Study the drawing (mm; zero at the part's minimum x, y, z) and answer. Coordinates: 2 decimals unless noted, no trailing zeros. Order: outer loops, then holes, each group sorted by start corner. A loop starts at its lowest first (then second) coordinate and runs counter-clockwise, first axis right, second up. Notation, with made-up numbers: (35, 80) -> (65, 80) arc R26 ccw to (65, 116) -> close; hole circle Ø1 at (10.25, -4.75). An arc over 180 degrees is marked (long way). Answer as CSV lines item,"result". Start each with the question number.
Item 1: Section C-C (x = 115) is taken. Write down the section's boundary in (y, z) (1 decimal).
Item 2: Straight lines are drawn through the part: L1, parallel to X at y = 15, z = 3.5; L2, parallel to Y at x = 127.5, z = 1.55 (1 decimal). For each, find the intervals that lie inside material, in ascending order.
Item 3: Section B-B (y = 126) is taken. Write down the section's boundary in (x, z).
Item 4: Each of these flat-tipped pins is pushed along its axis until it touches: pin 1 Ø1.2 at (y, z) = (3, 2.5) entering from +X; pin 2 Ø2 at (x, z) = (173.5, 3) entering from -Y (1 decimal); pin 3 Ø1.3 at (y, z) = (28.5, 3) entering from -X. Where does it stop, or does it pass through?
Item 5: Section A-A (z = 1.5) is taken. Write down the section's boundary in (x, y) (1 decimal), then the cut area to 3 significant figures.
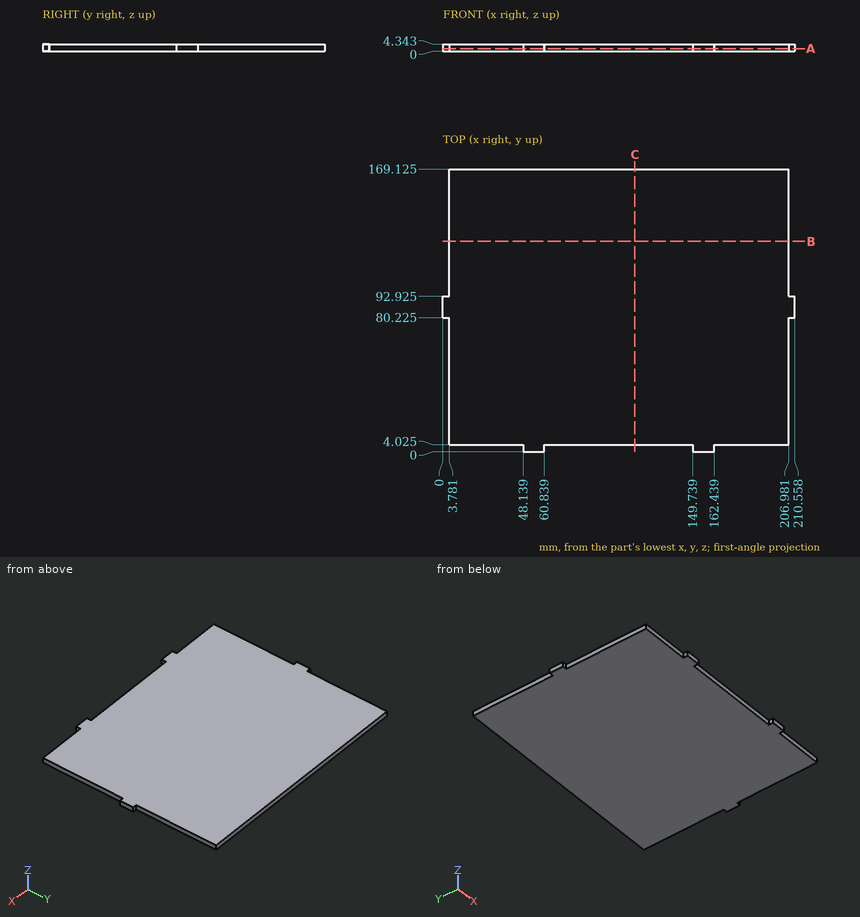
Checked values:
1,outline,"(4, 0) -> (169.1, 0) -> (169.1, 4.3) -> (4, 4.3) -> close"
2,L1,"x = 3.78 to 206.98"
2,L2,"y = 4 to 169.1"
3,outline,"(3.78, 0) -> (206.98, 0) -> (206.98, 4.34) -> (3.78, 4.34) -> close"
4,pin 1,"stops at x = 162.44"
4,pin 2,"stops at y = 4"
4,pin 3,"stops at x = 3.78"
5,outline,"(0, 80.2) -> (3.8, 80.2) -> (3.8, 4) -> (48.1, 4) -> (48.1, 0) -> (60.8, 0) -> (60.8, 4) -> (149.7, 4) -> (149.7, 0) -> (162.4, 0) -> (162.4, 4) -> (207, 4) -> (207, 80.2) -> (210.6, 80.2) -> (210.6, 92.9) -> (207, 92.9) -> (207, 169.1) -> (3.8, 169.1) -> (3.8, 92.9) -> (0, 92.9) -> close"
5,area,"33,700 mm^2"
